Design review of the part built by this model. Coordinates are the model's own, in mm. Face numbers are marked on the shaded views. A direction names the side the tool comes from. Give positions to 0.01 mm unless a question says otherwise; leave off trailing zeros. Write each loop counter-clockwise with the first axis right and the second up, starting at its lowest first coordinate (ties: lowest second). Pieces come first, ordered by that corner, then holes. Notation, with made-up numbers: (-34, 40) -> (-12, 40) arc R25 ccw to (-12, 67) -> close; hole circle Ø3 at (-25.5, 57.25). An arc over 180 degrees is marked (long way). Answer as a JSON object with one key per item and string values.
```python
from build123d import *

# Parameters (mm, degrees)
F0_R        = 185
F1_DEPTH    = 25
F2_R        = 22.5
F2_R_2      = 20
F3_DEPTH    = 40
F2_R_3      = 10
F2_R_4      = 7.5
F4_DEPTH    = 36
F3_FACE_R   = 22.5
F3_FACE_R_2 = 20
F5_DEPTH    = 5
F6_R        = 27.5
F6_R_2      = 20
F7_DEPTH    = 5
F8_R        = 15
F8_R_2      = 7.5
F9_DEPTH    = 5


with BuildPart() as f1:
    # F0 (on Top) → F1 (new body)
    with BuildSketch(Plane.XY):
        Circle(F0_R)
    extrude(amount=F1_DEPTH)

    # F2 (on face) → F3 (join)
    with BuildSketch(Plane.XY.offset(25)):
        Circle(F2_R)
        Circle(F2_R_2, mode=Mode.SUBTRACT)
        with Locations((120, 0)):
            Circle(F2_R)
        with Locations((120, 0)):
            Circle(F2_R_2, mode=Mode.SUBTRACT)
    extrude(amount=F3_DEPTH)

    # F2 (on face) → F4 (join)
    with BuildSketch(Plane.XY.offset(25)):
        with Locations((120, 0)):
            Circle(F2_R)
        with Locations((120, 0)):
            Circle(F2_R_2, mode=Mode.SUBTRACT)
        Circle(F2_R)
        Circle(F2_R_2, mode=Mode.SUBTRACT)
        with Locations((-135, 0)):
            Circle(F2_R_3)
        with Locations((-135, 0)):
            Circle(F2_R_4, mode=Mode.SUBTRACT)
    extrude(amount=F4_DEPTH)

    # F3_face (on face) → F5 (join)
    with BuildSketch(Plane.XY.offset(65)):
        Circle(F3_FACE_R)
        Circle(F3_FACE_R_2, mode=Mode.SUBTRACT)
        with Locations((120, 0)):
            Circle(F3_FACE_R)
        with Locations((120, 0)):
            Circle(F3_FACE_R_2, mode=Mode.SUBTRACT)
    extrude(amount=F5_DEPTH)

    # F6 (on face) → F7 (join)
    with BuildSketch(Plane.XY.offset(70)):
        with Locations((120, 0)):
            Circle(F6_R)
        with Locations((120, 0)):
            Circle(F6_R_2, mode=Mode.SUBTRACT)
        Circle(F6_R)
        Circle(F6_R_2, mode=Mode.SUBTRACT)
    extrude(amount=-F7_DEPTH)

    # F8 (on face) → F9 (join)
    with BuildSketch(Plane.XY.offset(61)):
        with Locations((-135, 0)):
            Circle(F8_R)
        with Locations((-135, 0)):
            Circle(F8_R_2, mode=Mode.SUBTRACT)
    extrude(amount=-F9_DEPTH)


solid = f1.part
```
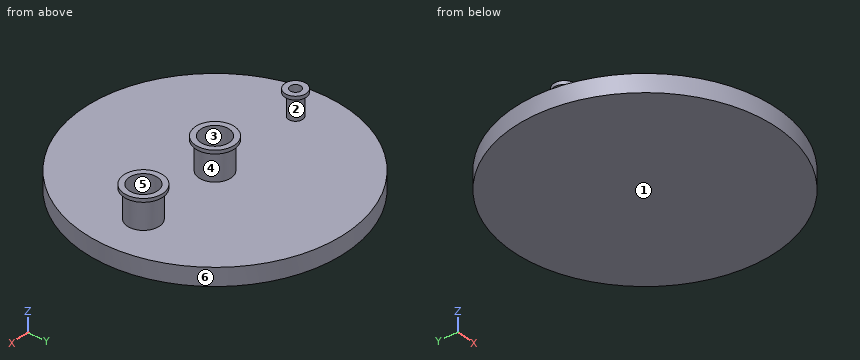
(1) We need section C-C, the plane z = 18.5. State the section outline as (x, y) points, then the cut area to 3 significant figures.
Here are the results:
{"outline": "circle Ø370 at (0, 0)", "area": "108,000 mm²"}
(2) Clearance check with flat-ended pins moving along their axes: pin 1 (4 mm diameter, centred on x = -30.5, y = 136.5, fed in from +Z); pin 2 (12 mm diameter, centred on x = 87.5, z = 27, fed in from +Y); pin 3 (1.5 mm diameter, centred on x = 141.5, z = 17.5, fed in from -Y). State where each tip first meets the part, or that it passes through.
Here are the results:
{"pin 1": "stops at z = 25", "pin 2": "stops at y = 165.91", "pin 3": "stops at y = -120.06"}
(3) For line 1 along X through (y, z) = (13.5, 52.5); line 2 along Z through (x, y) = (68, 79.5); line 3 along X through (y, z) = (103, 8), list the stretches that pass through material, from the lowest coordinate up.
Here are the results:
{"line 1": "x = -18 to -14.76, 14.76 to 18, 102 to 105.24, 134.76 to 138", "line 2": "z = 0 to 25", "line 3": "x = -153.67 to 153.67"}
(4) For the marked faces 4, 5 and 6, list the 3-axis set-ups (+Z, -Z, +X, -X, +Y, -Y) from which the entire face can be reached by the end or side of a thin tool; tool diameter is ignored.
Here are the results:
{"face 4": "none", "face 5": "+Z", "face 6": "+Z, -Z"}
(5) The part is to be moulded in two halves that separate along Z. For the marked faces 1, 2 and 3, say which applies: +Z half, -Z half, draft (parallel to the pull), parting line (faces both ways), or undercut.
Here are the results:
{"face 1": "-Z half", "face 2": "undercut", "face 3": "draft"}
(6) We need section B-B, the plane x = 0. State the section outline as (y, z) points, then the cut area to 4 significant figures.
Here are the results:
{"outline": "(-185, 0) -> (185, 0) -> (185, 25) -> (22.5, 25) -> (22.5, 65) -> (27.5, 65) -> (27.5, 70) -> (20, 70) -> (20, 25) -> (-20, 25) -> (-20, 70) -> (-27.5, 70) -> (-27.5, 65) -> (-22.5, 65) -> (-22.5, 25) -> (-185, 25) -> close", "area": "9,525 mm²"}
(7) We need section A-A, the plane z = 44. State the section outline as (x, y) points, then the cut area to 3 significant figures.
Here are the results:
{"outline": "circle Ø20 at (-135, 0); circle Ø45 at (0, 0); circle Ø45 at (120, 0); hole circle Ø15 at (-135, 0); hole circle Ø40 at (0, 0); hole circle Ø40 at (120, 0)", "area": "805 mm²"}
(8) We need section D-D, the plane y = 147.5. State the section outline as (x, z) points, then the cut area to 3 significant figures.
Here are the results:
{"outline": "(-111.66, 0) -> (111.66, 0) -> (111.66, 25) -> (-111.66, 25) -> close", "area": "5,580 mm²"}
